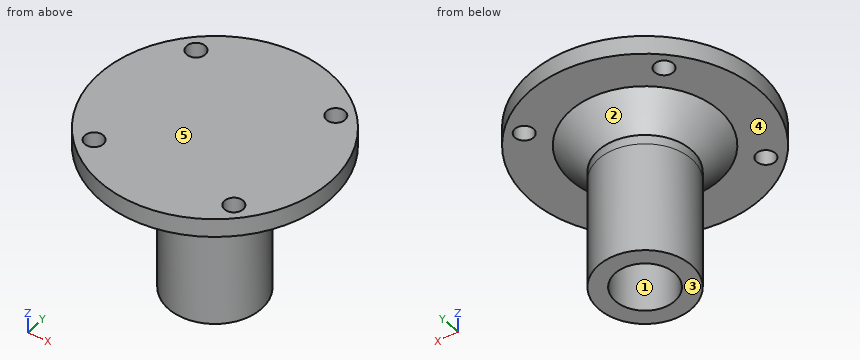
from build123d import *

# Parameters (mm, degrees)
SZKIC1_R                    = 12.5
SZKIC1_R_2                  = 8
DODANIE_WYCI_GNI_CIE1_DEPTH = 30
SZKIC2_R                    = 20
DODANIE_WYCI_GNI_CIE3_DEPTH = 10
SZKIC3_R                    = 31
DODANIE_WYCI_GNI_CIE4_DEPTH = 5
SFAZOWANIE1_SIZE            = 10
OTWORY_USTALAJ_CE_5_0MM1_D  = 5


with BuildPart() as part:
    # Szkic1 → Dodanie-wyciągnięcie1 (new body)
    with BuildSketch(Plane.XY):
        Circle(SZKIC1_R)
        Circle(SZKIC1_R_2, mode=Mode.SUBTRACT)
    extrude(amount=DODANIE_WYCI_GNI_CIE1_DEPTH)

    # Szkic2 → Dodanie-wyciągnięcie3 (add)
    with BuildSketch(Plane.XY.offset(30)):
        Circle(SZKIC2_R)
    extrude(amount=DODANIE_WYCI_GNI_CIE3_DEPTH)

    # Szkic3 → Dodanie-wyciągnięcie4 (add)
    with BuildSketch(Plane.XY.offset(40)):
        Circle(SZKIC3_R)
    extrude(amount=DODANIE_WYCI_GNI_CIE4_DEPTH)

    # Sfazowanie1
    # the kernel refuses this chamfer: 10 mm, written as the material it takes off along each edge
    with BuildSketch(Plane(origin=(0, 0, 30), x_dir=(1, 0, 0), z_dir=(0, -1, 0))) as sfazowanie1_piece_1_section:
        Polygon((20, SFAZOWANIE1_SIZE), (20 - SFAZOWANIE1_SIZE, 0), (20, 0), align=None)
    sfazowanie1_piece_1 = revolve(axis=Axis((0, 0, 30), (0, 0, 1)), mode=Mode.PRIVATE)
    sfazowanie1_piece_1 = split(sfazowanie1_piece_1, bisect_by=Plane(origin=(-16.374530577, 0, 40), z_dir=(0, 0, -1)), keep=Keep.TOP, mode=Mode.PRIVATE)
    sfazowanie1_piece_1 = sfazowanie1_piece_1 - Plane(origin=(0, 0, 36.125469423), x_dir=(1, 0, 0), z_dir=(0, 0, -1)) * Cylinder(12.5, 80, mode=Mode.PRIVATE)
    add(sfazowanie1_piece_1, mode=Mode.SUBTRACT)

    # Otwory ustalające Ø5.0mm1 (through all)
    with Locations(Plane(origin=(-18.74, 18.74, 45), x_dir=(1, 0, 0), z_dir=(0, 0, 1))):
        with Locations((0, 0), (37.48, 0), (37.48, -37.48), (0, -37.48)):
            Hole(OTWORY_USTALAJ_CE_5_0MM1_D / 2)


solid = part.part
Build history of the part. All positions in model axes, mm. Face numbers are marked on the shaded views. A direction names the side the tool comes from. Give positions to 0.01 mm unless a question says otherwise; leave off trailing zeros. Loops run counter-clockwise (first coordinate to the right, second up) from the corner with the lowest first, then second, coordinate; pieces in that order, holes last. Notation, with made-up numbers: (22.5, 78) - (50.5, 78) arc R13 ccw to (50.5, 89) - close; hole circle Ø8 at (19.5, -8.5). An arc over 180 degrees is marked (long way). Write item = value, one per line. Start each with the question number.
1) Band-saw the part on A-A on z = 12. Give the cut face in (x, y), plus the area to 3 significant figures.
2) Pull direction X, two halves, no side cores. Call the marked faces 1, 2 and 3: +X half, -X half, draft (parallel to the pull), parting line (faces both ways), or undercut.
3) Band-saw the part on B-B on x = 0. Give the cut face in (y, z), plus the area to 3 significant figures.
4) Drop flat-ended pins along their axis: pin 1 Ø4 at (y, z) = (-17, 39.5) entering from +X; pin 2 Ø1 at (y, z) = (0, 8) entering from +X; pin 3 Ø12 at (x, y) = (3.5, 19.5) entering from -Z; pin 4 Ø4 at (x, y) = (18.74, 18.74) entering from +Z. Give the stop position or say it passes through.
5) Probe probe 1 along Y at (x, z) = (-18.74, 42.2); probe 2 along Z at (x, y) = (-2.5, -27.5); probe 3 along X at (y, z) = (0.5, 30.5). List the from-to ranges inside material, lowest first. Write a range as from..to.
6) Band-saw the part on C-C on y = 18.74. Count the separate pieces of the cut face and the enclosed holes in it, plus the area to 3 significant figures.
7) Tool access for the marked faces 4 and 5: list every direction of +Z, -Z, +X, -X, +Y, -Y with a clear straight run to the whole face (end or side of a thin tool).
Final values:
q1.outline = circle Ø25 at (0, 0); hole circle Ø16 at (0, 0)
q1.area = 290 mm²
q2.face_1 = undercut
q2.face_2 = parting line
q2.face_3 = draft
q3.outline = (-31, 40) - (-20, 40) - (-12.5, 32.5) - (-12.5, 0) - (-8, 0) - (-8, 30) - (8, 30) - (8, 0) - (12.5, 0) - (12.5, 32.5) - (20, 40) - (31, 40) - (31, 45) - (-31, 45) - close
q3.area = 886 mm²
q4.pin_1 = 27.09
q4.pin_2 = 12.5
q4.pin_3 = 33.81
q4.pin_4 = through
q5.probe_1 = -24.69..-21.24, -16.24..16.24, 21.24..24.69
q5.probe_2 = 40..45
q5.probe_3 = -12.49..12.49
q6.separate_pieces = 3
q6.enclosed_holes = 0
q6.area = 209 mm²
q7.face_4 = -Z
q7.face_5 = +Z, +X, -X, +Y, -Y
